Autodesk Inventor part; units mm, degrees
ref_plane "YZ Plane" through (0, 0, 0) normal (1, 0, 0) x (0, 1, 0)
ref_plane "XZ Plane" through (0, 0, 0) normal (0, 1, 0) x (-1, 0, 0)
ref_plane "XY Plane" through (0, 0, 0) normal (0, 0, 1) x (1, 0, 0)
sketch "スケッチ1" plane through (0, 0, 0) normal (0, 0, 1) x (1, 0, 0)
  line L0 (5, -5) -> (-5, -5)
  line L1 (-5, -5) -> (-5, 5)
  line L2 (-5, 5) -> (5, 5)
  line L3 (5, 5) -> (5, -5)
  line L4 (5, -5) -> (-5, 5) construction
  line L5 (-5, -5) -> (5, 5) construction
  line L6 (4, 4) -> (-4, 4)
  line L7 (-4, 4) -> (-4, -4)
  line L8 (-4, -4) -> (4, -4)
  line L9 (4, -4) -> (4, 4)
  point P0 (0, 0)
  dimension "d0" = 10
  dimension "d1" = 10
  dimension "d2" = 1
extrude "押し出し1" add sketch "スケッチ1" along normal blind 300
sketch "スケッチ2" plane through (5, -5, 0) normal (1, 0, 0) x (0, 0, -1)
  line L0 (0, 0) -> (0, 10)
  line L1 (0, 10) -> (-300, 10)
  line L2 (-300, 0) -> (-300, 10)
  line L3 (0, 0) -> (-300, 0)
  line L4 (0, 5) -> (-300, 5)
  line L5 (-300, 0) -> (-300, 10)
  point P0 (-290, 5)
  point P1 (-176, 5)
  point P2 (-56, 5)
  point P3 (-10, 5)
  point P4 (-112, 5)
  point P5 (-243, 5)
  point P6 (-149.5, 5)
  dimension "d7" = 120
  dimension "d25" = 10
  dimension "d26" = 46
  dimension "d27" = 10
  dimension "d28" = 114
  dimension "d29" = 56
  dimension "d34" = 26.5
  dimension "d35" = 93.5
  dimension "d36" = 93.5
hole "穴1" at (5, 0, 290) at (5, 0, 176) at (5, 0, 56) at (5, 0, 10) at (5, 0, 112) at (5, 0, 243) direction (-1, 0, 0) diameter 3.3 end through all
sketch "スケッチ3" plane through (-5, 5, 0) normal (0, 1, 0) x (1, 0, 0)
  line L0 (10, 0) -> (0, 0)
  line L1 (0, 0) -> (0, -300)
  line L2 (10, -300) -> (0, -300)
  line L3 (10, 0) -> (10, -300)
  line L4 (5, -300) -> (5, 0)
  point P0 (5, -275)
  point P1 (5, -46)
  point P2 (5, -102)
  point P3 (5, -189)
  point P4 (5, -25)
  dimension "d17" = 25
  dimension "d30" = 46
  dimension "d31" = 56
  dimension "d32" = 87
  dimension "d33" = 25
hole "穴2" at (0, 5, 275) at (0, 5, 46) at (0, 5, 102) at (0, 5, 189) at (0, 5, 25) direction (0, -1, 0) diameter 3.3 end through all
properties part number "small_kaku_1010_200"
The model under review builds one solid part; all positions refer to its coordinate system, in mm. A direction names the side the tool comes from. Round coordinates to 2 decimals unless told otherwise and drop trailing zeros. Write each loop counter-clockwise with the first axis right and the second up, starting at its lowest first coordinate (ties: lowest second). Pieces come first, ordered by that corner, then holes.
(1) We need section A-A on z = 33.5. Give the boundary of the cut face in (x, y), and give its area (3 significant figures).
(2) Machinability: for faces 4 (the flat face through (-5, 0, 148)), 5 (the flat face through (-4, 0, 148)), which of the approach directions +Z, -Z, +X, -X, +Y, -Y give a long, thin tool a straight path to every point of the face, cutting with its end or side? Answer none if there is none.
(3) Wall thickness on L1, parallel to Y at x = -0.5, z = 54; L2, parallel to Z at x = 0, y = -4.75: over which ranges is each line inside the solid? List them lowest first.
(4) Insertion check: pin 1 (2.5 mm diameter, centred on x = 0, z = 25, fed in from -Y). The pin has a flat end and moves straight along its axis. Give the tip position at first contact, or say it passes through.
(5) We need section B-B on y = 0. Give the number of separate pieces and of enclosed holes in the cut face, and give its area (3 significant figures).
(6) Mouldability with a two-part tool opening along X and no side actions: class faces 1 (the flat face through (0, 4, 148)), 2 (the flat face through (-4.5, 0.1, 300)), 3 (the flat face through (5, 0, 148)) as +X half, -X half, draft (parallel to the pull), parting line (faces both ways), or undercut.
Findings below:
1. outline: (-5, -5) - (5, -5) - (5, 5) - (-5, 5) - close; hole (-4, -4) - (4, -4) - (4, 4) - (-4, 4) - close
1. area: 36.0 mm2
2. face 4: +Z, -Z, -X, +Y, -Y
2. face 5: +Z, -Z
3. L1: y = -5 to -4, 4 to 5
3. L2: z = 0 to 23.35, 26.65 to 44.35, 47.65 to 100.35, 103.65 to 187.35, 190.65 to 273.35, 276.65 to 300
4. pin 1: passes through
5. separate pieces: 14
5. enclosed holes: 0
5. area: 560 mm2
6. face 1: undercut
6. face 2: draft
6. face 3: +X half
